Autodesk Inventor part; units mm, degrees
ref_plane "YZ Plane" through (0, 0, 0) normal (1, 0, 0) x (0, 1, 0)
ref_plane "XZ Plane" through (0, 0, 0) normal (0, 1, 0) x (-1, 0, 0)
ref_plane "XY Plane" through (0, 0, 0) normal (0, 0, 1) x (1, 0, 0)
sketch "Base" plane through (0, 0, 0) normal (0, 0, 1) x (1, 0, 0)
  circle A0 centre (0, 0) radius 3.125
  circle A1 centre (0, 0) radius 12.7
  line L0 (0, 12.7) -> (60, 12.7)
  line L1 (60, 12.7) -> (60, -12.7)
  line L2 (60, -12.7) -> (0, -12.7)
  dimension "d0" = 6.25
  dimension "d1" = 25.4
  dimension "d2" = 60
extrude "Plate1" add sketch "Base" along normal blind 2
sketch "Sketch2" plane through (58, -12.7, 2) normal (1, 0, 0) x (0, 1, 0)
  line L0 (25.4, 0) -> (0, 0)
  line L1 (0, 0) -> (0, -20)
  line L2 (0, -20) -> (25.4, -20)
  line L3 (25.4, -20) -> (25.4, 0)
edge flange "MountFeature" height 20 angle 90 thickness 2 bend radius 2 thickness toward (1, 0, 0) relief tear relief width 2 relief depth 1 edges at (60, 0, 0) wall of the first edge with corners at (58, 12.7, 2) (58, -12.7, 2) (58, -12.7, -18) (58, 12.7, -18)
bend "Bend1"
corner "Corner1"
fillet "MountFilletsFeature" radius 4 2 edges at (59, -12.7, -18) (59, 12.7, -18)
sketch "HubMountHoles" plane through (0, 0, 2) normal (0, 0, 1) x (1, 0, 0)
  circle A0 centre (0, 9.35) radius 1.25
  circle A1 centre (8.0973, 4.675) radius 1.25
  circle A2 centre (8.0973, -4.675) radius 1.25
  circle A3 centre (0, -9.35) radius 1.25
  circle A4 centre (-8.0973, -4.675) radius 1.25
  circle A5 centre (-8.0973, 4.675) radius 1.25
  point P0 (0, 0)
extrude "HubMountHolesFeature" cut sketch "HubMountHoles" against normal blind 2
sketch "PotMountHoles" plane through (0, 0, 2) normal (0, 0, 1) x (1, 0, 0)
  arc A0 (2.191, 15.5897) -> (-4.4715, 15.0972) centre (0.0082, -0.192) ccw
  arc A1 (-4.4715, 15.0972) -> (-3.8455, 12.9843) centre (-4.1585, 14.0408) ccw
  arc A2 (1.887, 13.4273) -> (-3.8455, 12.9843) centre (0.0734, -0.4153) ccw
  arc A3 (1.887, 13.4273) -> (2.191, 15.5897) centre (2.0448, 14.5077) ccw
  circle A4 centre (5.0089, 13.7622) radius 0.75
  circle A5 centre (-5.0089, -13.7614) radius 0.75
  arc A6 (-1.8863, -13.4212) -> (-2.1909, -15.5889) centre (-2.0386, -14.505) ccw
  arc A7 (-1.8863, -13.4212) -> (3.8453, -12.9835) centre (-0.0533, 0.3202) ccw
  arc A8 (-2.1909, -15.5889) -> (4.5487, -15.0702) centre (-0.0101, 0.1221) ccw
  arc A9 (4.5487, -15.0702) -> (3.8453, -12.9835) centre (4.1564, -14.0405) ccw
  circle A10 centre (0, 0) radius 3.125
  circle A11 centre (0, 0) radius 17
  circle A12 centre (-8.0973, 4.675) radius 1.25
  circle A13 centre (0, 9.35) radius 1.25
  circle A14 centre (8.0973, 4.675) radius 1.25
  circle A15 centre (8.0973, -4.675) radius 1.25
  circle A16 centre (0, -9.35) radius 1.25
  circle A17 centre (-8.0973, -4.675) radius 1.25
  dimension "d17" = 34
sheet face with bend "PotMountHolesFeature" sketch "PotMountHoles" thickness 2 toward (0, 0, -1) bend radius 2
bend "Bend3"
sketch "Sketch5" plane through (60, -12.7, -2) normal (1, 0, 0) x (0, 0, -1)
  line L0 (0, 25.4) -> (12, 25.4) construction
  line L1 (12, 0) -> (0, 0) construction
  line L2 (10, 25.4) -> (10, 0) construction
  circle A0 centre (10, 19.4) radius 3
  circle A1 centre (10, 6) radius 3
  line L3 (16, 21.4) -> (16, 4)
  point P0 (-2, 12.7)
  dimension "d28" = 6
  dimension "d29" = 6
  dimension "d30" = 6
  dimension "d31" = 6
  dimension "d32" = 6
extrude "Cut2" cut sketch "Sketch5" against normal blind 2
equation "\"d15\" = Thickness"
equation "\"d33\" = Thickness"
equation "\"d3\" = Thickness"
equation "\"d4\" = BendReliefWidth"
equation "\"d5\" = BendReliefDepth"
equation "\"d6\" = MinimumRemnant"
equation "\"d7\" = TransitionRadius"
equation "\"d10\" = BendRadius"
equation "\"d11\" = CornerReliefSize"
equation "\"d12\" = GapSize"
equation "\"d13\" = JacobiRadiusSize"
equation "\"d23\" = BendRadius"
equation "\"d24\" = BendReliefWidth"
equation "\"d26\" = MinimumRemnant"
equation "\"d25\" = BendReliefDepth"
equation "\"d27\" = TransitionRadius"
equation "\"BendRadius\" = Thickness"
equation "\"BendReliefWidth\" = Thickness"
equation "\"BendReliefDepth\" = 0.5 * Thickness"
equation "\"CornerReliefSize\" = 4 * Thickness"
equation "\"MinimumRemnant\" = 2 * Thickness"
equation "\"TransitionRadius\" = BendRadius"
equation "\"JacobiRadiusSize\" = BendRadius"
equation "\"GapSize\" = Thickness"
properties part number "NeckPotentiometerBracket"
Can you work these out from the model? Positions are in its coordinate system, mm. A direction names the side the tool comes from. Give positions to 0.01 mm unless a question says otherwise; leave off trailing zeros. Loops run counter-clockwise (first coordinate to the right, second up) from the corner with the lowest first, then second, coordinate; pieces in that order, holes last. Notation, with made-up numbers: (48, 25.5) -> (106, 25.5) arc R25 cw to (106, 46.5) -> close; hole circle Ø3 at (21, 84.25). An arc over 180 degrees is marked (long way). Return JSON: item names as keys, results as strings.
Q1. I want a section at B-B, the plane z = -12. List the corners of the cut face in (x, y) for me.
Checks:
{"outline": "(58, -12.7) -> (60, -12.7) -> (60, -9.7) -> (58, -9.7) -> close; (58, -3.7) -> (60, -3.7) -> (60, 3.7) -> (58, 3.7) -> close; (58, 9.7) -> (60, 9.7) -> (60, 12.7) -> (58, 12.7) -> close"}
Q2. I want a section at C-C, the plane x = 0. List the corners of the cut face in (y, z) for me (3 decimals).
Checks:
{"outline": "(-17, 0) -> (-15.74, 0) -> (-15.74, 2) -> (-17, 2) -> close; (-13.543, 0) -> (-10.6, 0) -> (-10.6, 2) -> (-13.543, 2) -> close; (-8.1, 0) -> (-3.125, 0) -> (-3.125, 2) -> (-8.1, 2) -> close; (3.125, 0) -> (8.1, 0) -> (8.1, 2) -> (3.125, 2) -> close; (10.6, 0) -> (13.545, 0) -> (13.545, 2) -> (10.6, 2) -> close; (15.74, 0) -> (17, 0) -> (17, 2) -> (15.74, 2) -> close"}
Q3. I need wall thicknesses on probe 1 along Y at (x, z) = (58.4, -12); probe 2 along Z at (x, y) = (-13, -2); probe 3 along X at (y, z) = (11.5, -15.5). Which ranges of each line are inside material? Lowest first, please.
Checks:
{"probe 1": "y = -12.7 to -9.7, -3.7 to 3.7, 9.7 to 12.7", "probe 2": "z = 0 to 2", "probe 3": "x = 58 to 60"}
Q4. I want a section at D-D, the plane y = 6.7. List the corners of the cut face in (x, z) for me.
Checks:
{"outline": "(-15.62, 0) -> (56, 0) arc R2 cw to (58, -2) -> (58, -9) -> (60, -9) -> (60, -2) arc R4 ccw to (56, 2) -> (-15.62, 2) -> close; (58, -18) -> (60, -18) -> (60, -15) -> (58, -15) -> close"}
Q5. For pin 1 Ø8 at (y, z) = (7.5, -13) entering from -X; pin 2 Ø9.5 at (y, z) = (6.7, -12) entering from +X; pin 3 Ø3 at (x, y) = (8.1, -4.68) entering from -Z, each with a flat end and sliding along its axis, tell me the tip position at first contact or that it passes through.
Checks:
{"pin 1": "stops at x = 58", "pin 2": "stops at x = 60", "pin 3": "stops at z = 0"}
Q6. I want a section at A-A, the plane y = 0. List the corners of the cut face in (x, z) for me (3 decimals).
Checks:
{"outline": "(-17, 0) -> (-3.125, 0) -> (-3.125, 2) -> (-17, 2) -> close; (3.125, 0) -> (56, 0) arc R2 cw to (58, -2) -> (58, -18) -> (60, -18) -> (60, -2) arc R4 ccw to (56, 2) -> (3.125, 2) -> close"}
Q7. We'd pull the mould along Y, two halves only. Please class faces 1 (the face through (19, 0, 2)), 2 (the face through (-0.27, 8.13, 1.01)), 3 (the face through (41, -12.7, 1)): released by +Y, released by -Y, zero draft, split by the parting line, or undercut.
Checks:
{"face 1": "zero draft", "face 2": "undercut", "face 3": "released by -Y"}
Q8. On a 3-axis mill with a long thin cutter (end or side, diameter ignored), from which of +Z, -Z, +X, -X, +Y, -Y can I reach the whole of each face in a straight line? I mean faces 4 (the face through (59, 0, -18)), 5 (the face through (-1.1, 15.7, 1)), 6 (the face through (58, 0, -10)). Say none if no direction works.
Checks:
{"face 4": "-Z, +X, -X, +Y, -Y", "face 5": "+Z, -Z", "face 6": "-Z, -X, +Y, -Y"}
